Could you check a few things on this drawing? It's one solid part, dimensions in mm from its lowest x, y, z. A direction names the side the tool comes from. Round coordinates to 2 decimals unless told otherwise and drop trailing zeros. Loops run counter-clockwise (first coordinate to the right, second up) from the corner with the lowest first, then second, coordinate; pieces in that order, holes last. Notation, with made-up numbers: M 30.5,47.5 L 37.5,47.5 A23 cw 37.5,69.5 Z; hole C 36,-23 d8. An arc over 180 degrees is marked long. Answer as CSV lines item,"result".
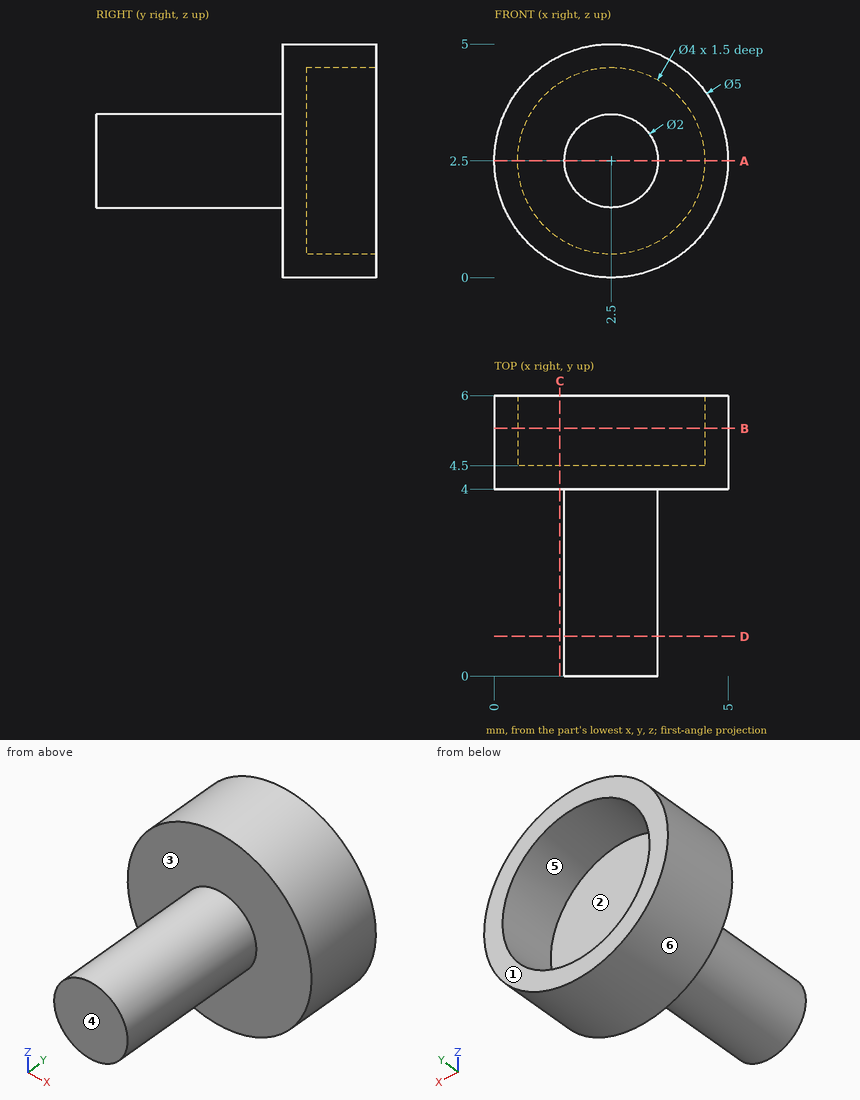
Item 1: If we section it at A-A on z = 2.5: Write out the boundary of the cut face in (x, y), then the cut area to 3 significant figures.
Output:
outline,"M 0,4 L 1.5,4 L 1.5,0 L 3.5,0 L 3.5,4 L 5,4 L 5,6 L 4.5,6 L 4.5,4.5 L 0.5,4.5 L 0.5,6 L 0,6 Z"
area,"12.0 mm2"
Item 2: If we section it at B-B on y = 5.3: Write out the boundary of the cut face in (x, z), then the cut area to 3 significant figures.
Output:
outline,"C 2.5,2.5 d5; hole C 2.5,2.5 d4"
area,"7.07 mm2"
Item 3: We'd pull the mould along X, two halves only. Please class the marked faces 4, 5 and 6: released by +X, released by -X, zero draft, split by the parting line, or undercut.
Output:
face 4,"zero draft"
face 5,"undercut"
face 6,"split by the parting line"
Item 4: If I drill on line 1 along X through (y, z) = (5.2, 2.5); line 2 along Y through (x, z) = (0.55, 1.7); line 3 along Y through (x, z) = (4.1, 3.15), over which ranges is the centre line in solid material (lowest first)? Write a range as from..to.
Output:
line 1,"x = 0..0.5, 4.5..5"
line 2,"y = 4..6"
line 3,"y = 4..4.5"
Item 5: If we section it at C-C on x = 1.4: Write out the boundary of the cut face in (y, z) (3 decimals), then the cut area to 3 significant figures.
Output:
outline,"M 4,0.255 L 6,0.255 L 6,0.83 L 4.5,0.83 L 4.5,4.17 L 6,4.17 L 6,4.745 L 4,4.745 Z"
area,"3.97 mm2"
Item 6: On a 3-axis mill with a long thin cutter (end or side, diameter ignored), from which of +Z, -Z, +X, -X, +Y, -Y can I reach the whole of each face in a straight line? I mean the marked faces 1, 2 and 3. Say none if no direction works.
Output:
face 1,"+Z, -Z, +X, -X, +Y"
face 2,"+Y"
face 3,"-Y"
Item 7: If we section it at D-D on y = 0.85: Write out the boundary of the cut face in (x, z), then the cut area to 3 significant figures.
Output:
outline,"C 2.5,2.5 d2"
area,"3.14 mm2"
